Check sheet for the modelled part. Datum: model origin and axes. Units: mm. A direction names the side the tool comes from. Round coordinates to 2 decimals unless told otherwise and drop trailing zeros. Write each loop counter-clockwise with the first axis right and the second up, starting at its lowest first coordinate (ties: lowest second). Pieces come first, ordered by that corner, then holes.
Item 1: Cross-section at C-C on y = 30. Enter the section's corners in (x, z).
Item 2: Cross-section at B-B on z = 19.5. Enter the section's corners in (x, y) (3 decimals), plus the area to 3 significant figures.
Item 3: Cross-section at D-D on y = 17. Enter the section's corners in (x, z).
Item 4: Tool access check on faces 1 (the cylindrical face through (1.359, 7.114, 28.27)), 2 (the flat face through (-11.926, 52, 5)), 3 (the flat face through (1, 14, 0)), 4 (the cylindrical face through (-12.206, 52.144, 0.123)). Record the directions out of +Z, -Z, +X, -X, +Y, -Y that give a thin tool (end or side, any length) a straight path to the whole face; none if there is none.
Item 5: Cross-section at A-A on y = 51. Enter the section's corners in (x, z), plus the area to 3 significant figures.
Item 6: Release check for a two-part mould opening along Y. For faces 5 (the flat face through (1, 57, 12.243)), 6 (the cylindrical face through (-12.29, 52.25, 11.01)), 7 (the flat face through (1, 6.35, 9)), 8 (the flat face through (-3, 94.107, 1)) record: +Y half, -Y half, draft (parallel to the pull), parting line (faces both ways), or undercut.
Item 7: Go/stop test with flat-tipped pins: pin 1 Ø3 at (x, y) = (-3, 74) entering from +Z; pin 2 Ø4 at (x, y) = (-5.5, 78.5) entering from -Z; pin 3 Ø3 at (x, y) = (-1, 73) entering from -Z. Record where each tip stops, or that it passes through.
Item 8: Material ranges on line 1 (Y direction, x = 10.5, z = 11.5) (3 decimals); line 2 (Y direction, x = -7.75, z = -5.5); line 3 (Y direction, x = -11.5, z = -4), recorded low to high.
from build123d import *

# Parameters (mm, degrees)
SKETCH1_W               = 29.532117275
SKETCH1_H               = 16.294493356
BOSS_EXTRUDE1_DEPTH     = 6.35
BOSS_EXTRUDE2_DEPTH     = 82.55
SKETCH2_W               = 29.532117275
SKETCH2_H               = 16.294493356
CUT_EXTRUDE1_DEPTH      = 3.175
SKETCH4_W               = 29.532117275
SKETCH4_H               = 12.7
BOSS_EXTRUDE3_DEPTH     = 3.175
SKETCH7_W               = 36.710026843
SKETCH7_H               = 7.62
CUT_EXTRUDE4_DEPTH      = 13.589
SKETCH8_W               = 36.710026843
SKETCH8_H               = 7.62
CUT_EXTRUDE5_DEPTH      = 13.589
SKETCH9_W               = 29.532117275
SKETCH9_H               = 76.2
SKETCH9_W_2             = 22.877365929
SKETCH9_H_2             = 7.62
BOSS_EXTRUDE5_DEPTH     = 12.2428
CUT_EXTRUDE6_DEPTH      = 95.918198917
CUT_EXTRUDE6_DEPTH_BACK = 95.918198917
SKETCH10_R              = 2.4892
FILLET2_R               = 2.54
FILLET3_R               = 2.54


with BuildPart() as part:
    # Sketch1 → Boss-Extrude1 (new body)
    with BuildSketch(Plane(origin=(0, 0, 0), x_dir=(1, 0, 0), z_dir=(0, 1, 0))):
        Polygon((16.296436439, 0), (-13.235680836, 21.805506644), (-13.235680836, 0), align=None)
        with Locations((1.530377802, -8.147246678)):
            Rectangle(SKETCH1_W, SKETCH1_H)
    extrude(amount=BOSS_EXTRUDE1_DEPTH)

    # Sketch1<3> → Boss-Extrude2 (add)
    with BuildSketch(Plane(origin=(0, 0, 0), x_dir=(1, 0, 0), z_dir=(0, 1, 0))):
        Polygon((16.296436439, 0), (-13.235680836, 21.805506644), (-13.235680836, 0), align=None)
    extrude(amount=-BOSS_EXTRUDE2_DEPTH)

    # Sketch2 → Cut-Extrude1 (cut)
    with BuildSketch(Plane(origin=(0, 0, 0), x_dir=(-1, 0, 0), z_dir=(0, -1, 0))):
        with Locations((-1.530377802, -8.147246678)):
            Rectangle(SKETCH2_W, SKETCH2_H)
    extrude(amount=-CUT_EXTRUDE1_DEPTH, mode=Mode.SUBTRACT)

    # Sketch4 → Boss-Extrude3 (add)
    with BuildSketch(Plane(origin=(0, 6.35, 0), x_dir=(1, 0, 0), z_dir=(0, 1, 0))):
        with Locations((1.530377802, -22.644493356)):
            Rectangle(SKETCH4_W, SKETCH4_H)
    extrude(amount=-BOSS_EXTRUDE3_DEPTH)

    # Sketch7 → Cut-Extrude4 (cut)
    with BuildSketch(Plane(origin=(3.863909533, 0, -5.233055638), x_dir=(-0.804470053980136, 0, -0.5939932089251503), z_dir=(0.5939932089251503, 0, -0.804470053980136))):
        with Locations((5.24501832, -77.597)):
            Rectangle(SKETCH7_W, SKETCH7_H)
    extrude(amount=-CUT_EXTRUDE4_DEPTH, mode=Mode.SUBTRACT)

    # Sketch8 → Cut-Extrude5 (cut)
    with BuildSketch(Plane(origin=(3.863909533, 0, -5.233055638), x_dir=(-0.804470053980136, 0, -0.5939932089251503), z_dir=(0.5939932089251503, 0, -0.804470053980136))):
        with Locations((5.24501832, -39.497)):
            Rectangle(SKETCH8_W, SKETCH8_H)
    extrude(amount=-CUT_EXTRUDE5_DEPTH, mode=Mode.SUBTRACT)

    # Sketch9 → Boss-Extrude5 (add)
    with BuildSketch(Plane.XY):
        with Locations((1.530377802, -44.45)):
            Rectangle(SKETCH9_W, SKETCH9_H)
        with Locations((-0.487425481, -77.597)):
            Rectangle(SKETCH9_W_2, SKETCH9_H_2, mode=Mode.SUBTRACT)
        with Locations((-0.487425481, -39.497)):
            Rectangle(SKETCH9_W_2, SKETCH9_H_2, mode=Mode.SUBTRACT)
    extrude(amount=BOSS_EXTRUDE5_DEPTH)

    # Sketch10 → Cut-Extrude6 (cut, two sides: drawn at the far end of the back side and taken through both)
    with BuildSketch(Plane(origin=(0, -82.55, 0), x_dir=(-1, 0, 0), z_dir=(0, -1, 0)).offset(-CUT_EXTRUDE6_DEPTH_BACK)):
        with Locations(Location((3.710680836, -4.6228, 0), (0, 0, 270))):
            Circle(SKETCH10_R)
    extrude(amount=CUT_EXTRUDE6_DEPTH + CUT_EXTRUDE6_DEPTH_BACK, mode=Mode.SUBTRACT)

    # Fillet2
    # the kernel refuses this fillet: 2.54 mm, written as the material it takes off along each edge
    with BuildSketch(Plane(origin=(-13.235680836, -95.13201822, -21.805506644), x_dir=(0.8044700539801357, 0, 0.5939932089251506), z_dir=(0, 1, 0))) as fillet2_piece_1:
        with BuildLine():
            CenterArc((FILLET2_R * 1.98142019214, -FILLET2_R), FILLET2_R, 90, 126.440893479)
            Line((FILLET2_R * 1.17695013816, -FILLET2_R * 1.59399320893), (0, 0))
            Line((0, 0), (FILLET2_R * 1.98142019214, 0))
        make_face()
    extrude(amount=114.06403644, mode=Mode.SUBTRACT)
    with BuildSketch(Plane(origin=(-11.926108446, -81.407, 0), x_dir=(-0.8044700539801358, 0, -0.5939932089251506), z_dir=(0, 1, 0))) as fillet2_piece_2:
        with BuildLine():
            CenterArc((FILLET2_R * 0.504688507753, FILLET2_R), FILLET2_R, 216.440893479, 53.559106521)
            Line((-FILLET2_R * 0.299781546228, FILLET2_R * 0.406006791075), (0, 0))
            Line((0, 0), (FILLET2_R * 0.504688507753, 0))
        make_face()
    extrude(amount=7.62, mode=Mode.SUBTRACT)
    with BuildSketch(Plane(origin=(-11.926108446, -81.407, 12.2428), x_dir=(-1, 0, 0), z_dir=(0, 1, 0)), Plane(origin=(-11.926108446, -43.307, 12.2428), x_dir=(-1, 0, 0), z_dir=(0, 1, 0))) as fillet2_piece_3:
        with BuildLine():
            CenterArc((FILLET2_R, -FILLET2_R), FILLET2_R, 90, 90)
            Line((0, -FILLET2_R), (0, 0))
            Line((0, 0), (FILLET2_R, 0))
        make_face()
    extrude(amount=7.62, mode=Mode.SUBTRACT)
    with BuildSketch(Plane(origin=(-11.926108446, -35.687, 0), x_dir=(-0.8044700539801356, 0, -0.5939932089251507), z_dir=(0, -1, 0))) as fillet2_piece_4:
        with BuildLine():
            CenterArc((FILLET2_R * 0.504688507753, -FILLET2_R), FILLET2_R, 90, 53.559106521)
            Line((-FILLET2_R * 0.299781546228, -FILLET2_R * 0.406006791075), (0, 0))
            Line((0, 0), (FILLET2_R * 0.504688507753, 0))
        make_face()
    extrude(amount=7.62, mode=Mode.SUBTRACT)
    with BuildSketch(Plane(origin=(-13.235680836, 12.7, 28.994493356), x_dir=(0, 0, -1), z_dir=(0, -1, 0))) as fillet2_piece_5:
        with BuildLine():
            CenterArc((FILLET2_R, FILLET2_R), FILLET2_R, 180, 90)
            Line((0, FILLET2_R), (0, 0))
            Line((0, 0), (FILLET2_R, 0))
        make_face()
    extrude(amount=15.875, mode=Mode.SUBTRACT)
    with BuildSketch(Plane(origin=(16.296436439, 12.7, 28.994493356), x_dir=(0, 0, -1), z_dir=(0, -1, 0))) as fillet2_piece_6:
        with BuildLine():
            CenterArc((FILLET2_R, -FILLET2_R), FILLET2_R, 90, 90)
            Line((0, -FILLET2_R), (0, 0))
            Line((0, 0), (FILLET2_R, 0))
        make_face()
    extrude(amount=15.875, mode=Mode.SUBTRACT)

    # Fillet3
    fillet3_edges = [part.edges().sort_by_distance(p)[0] for p in [
        (-13.235680836, 6.35, 4.840897),
        (1.530377801, 6.35, 28.994493356),
        (16.296436439, 6.35, 13.227246678),
        (15.552487663, 6.35, 28.25054458),
        (-12.491732061, 6.35, 28.25054458),
        (-11.840100649, 6.35, -19.04027588),
        (3.554749177, 6.35, -9.408026646),
    ]]
    fillet(fillet3_edges, radius=FILLET3_R)


with BuildPart() as body_2:
    # Mirror1: mirrored copy
    add(part.part.mirror(Plane.ZX.offset(6.35)))


solid = body_2.part
Response values:
1. outline: (-13.24, -16.77) arc R2.54 ccw to (-9.19, -18.82) - (16.3, 0) - (16.3, 12.24) - (-13.24, 12.24) - close; hole circle Ø4.98 at (-3.71, 4.62)
2. outline: (-13.236, 8.89) arc R2.54 ccw to (-10.696, 6.35) - (13.756, 6.35) arc R2.54 ccw to (16.296, 8.89) - (16.296, 9.525) - (-13.236, 9.525) - close
2. area: 91.0 mm2
3. outline: (-13.24, -16.77) arc R2.54 ccw to (-9.19, -18.82) - (16.3, 0) - (-13.24, 0) - close
4. face 1: +Z, +X, -X, -Y
4. face 2: +Z
4. face 3: +Z, +X, -X
4. face 4: none
5. outline: (-13.24, -0.97) - (-12.96, -0.76) arc R2.54 ccw to (-11.93, 1.28) - (-11.93, 9.7) arc R2.54 ccw to (-13.24, 11.92) - close; (-13.05, -17.72) arc R2.54 ccw to (-9.19, -18.82) - (16.3, 0) - (16.3, 12.24) - (10.95, 12.24) - (10.95, 0) - close
5. area: 181 mm2
6. face 5: draft
6. face 6: undercut
6. face 7: -Y half
6. face 8: undercut
7. pin 1: stops at z = 12.24
7. pin 2: stops at z = -17.57
7. pin 3: stops at z = -13.88
8. line 1: y = 6.35 to 9.525, 19.05 to 48.387, 56.007 to 86.487, 94.107 to 95.25
8. line 2: y = 6.35 to 48.39, 56.01 to 86.49, 94.11 to 95.25
8. line 3: y = 6.48 to 48.39, 56.01 to 86.49, 94.11 to 95.25
